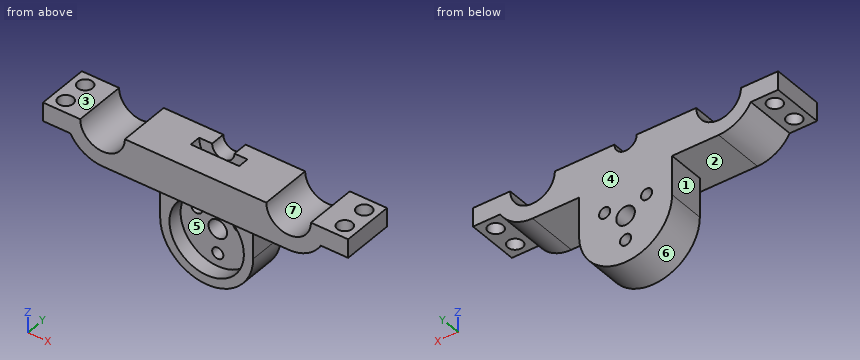
```python
from build123d import *

# Parameters (mm, degrees)
BOSS_EXTRUDE1_DEPTH     = 14
CUT_EXTRUDE1_DEPTH      = 45.463468151
CUT_EXTRUDE1_DEPTH_BACK = 45.463468151
SKETCH4_R               = 2
SKETCH5_W               = 9.30871577
SKETCH5_H               = 4.044371358
BOSS_EXTRUDE2_DEPTH     = 7
CUT_EXTRUDE2_START      = 1.5
SKETCH6_R               = 6.5
CUT_EXTRUDE2_DEPTH      = 1.5
BOSS_EXTRUDE3_DEPTH     = 10
SKETCH8_R               = 10
CUT_EXTRUDE3_DEPTH      = 4
SKETCH9_R               = 2.5
CUT_EXTRUDE4_DEPTH      = 54.235326617
SKETCH10_R              = 1.5
CUT_EXTRUDE5_DEPTH      = 54.235326617


with BuildPart() as part:
    # Sketch2 → Boss-Extrude1 (new body)
    with BuildSketch(Plane(origin=(0, 0, 0), x_dir=(1, 0, 0), z_dir=(0, 1, 0))):
        with BuildLine():
            Line((-3, 0), (-19, 0))
            ThreePointArc((-19, 0), (-25, 6), (-31, 0))
            Line((-31, 0), (-41, 0))
            Line((-41, 0), (-41, 5))
            Line((-41, 5), (-33.660254038, 5))
            ThreePointArc((-33.660254038, 5), (-30, 8.660254038), (-25, 10))
            Line((-25, 10), (25, 10))
            ThreePointArc((25, 10), (30, 8.660254038), (33.660254038, 5))
            Line((33.660254038, 5), (41, 5))
            Line((41, 5), (41, 0))
            Line((41, 0), (31, 0))
            ThreePointArc((31, 0), (25, 6), (19, 0))
            Line((19, 0), (3, 0))
            ThreePointArc((3, 0), (0, 3), (-3, 0))
        make_face()
    extrude(amount=BOSS_EXTRUDE1_DEPTH)

    # Sketch4 → Cut-Extrude1 (cut, two sides: drawn at the far end of the back side and taken through both)
    with BuildSketch(Plane.XY.offset(-CUT_EXTRUDE1_DEPTH_BACK)):
        with Locations((-37.5, 10.5)):
            Circle(SKETCH4_R)
        with Locations((-37.5, 3.5)):
            Circle(SKETCH4_R)
        with Locations((37.5, 10.5)):
            Circle(SKETCH4_R)
        with Locations((37.5, 3.5)):
            Circle(SKETCH4_R)
    extrude(amount=CUT_EXTRUDE1_DEPTH + CUT_EXTRUDE1_DEPTH_BACK, mode=Mode.SUBTRACT)

    # Sketch5 → Boss-Extrude2 (add)
    with BuildSketch(Plane.XZ):
        with Locations((-0.028958253, -2.022185679)):
            Rectangle(SKETCH5_W, SKETCH5_H)
    extrude(amount=-BOSS_EXTRUDE2_DEPTH)

    # Sketch6 → Cut-Extrude2 (cut, symmetric)
    with BuildSketch(Plane(origin=(0, 7, 0), x_dir=(1, 0, 0), z_dir=(0, 1, 0)).offset(CUT_EXTRUDE2_START)):
        Circle(SKETCH6_R)
    extrude(amount=CUT_EXTRUDE2_DEPTH, both=True, mode=Mode.SUBTRACT)

    # Sketch7 → Boss-Extrude3 (add)
    with BuildSketch(Plane(origin=(0, 14, 0), x_dir=(1, 0, 0), z_dir=(0, 1, 0))):
        with BuildLine():
            Line((-12.5, 20.5), (-12.5, 10))
            Line((-12.5, 10), (12.5, 10))
            Line((12.5, 10), (12.5, 20.5))
            ThreePointArc((12.5, 20.5), (0, 33), (-12.5, 20.5))
        make_face()
    extrude(amount=-BOSS_EXTRUDE3_DEPTH)

    # Sketch8 → Cut-Extrude3 (cut)
    with BuildSketch(Plane.XZ.offset(-4)):
        with Locations(Location((0, -20.5, 0), (0, 0, 270))):
            Circle(SKETCH8_R)
    extrude(amount=-CUT_EXTRUDE3_DEPTH, mode=Mode.SUBTRACT)

    # Sketch9 → Cut-Extrude4 (cut, through all)
    with BuildSketch(Plane.XZ.offset(-8)):
        with Locations(Location((0, -20.5, 0), (0, 0, 270))):
            Circle(SKETCH9_R)
    extrude(amount=-CUT_EXTRUDE4_DEPTH, mode=Mode.SUBTRACT)

    # Sketch10 → Cut-Extrude5 (cut, through all)
    with BuildSketch(Plane.XZ.offset(-8)):
        with Locations(Location((0, -27, 0), (0, 0, 270))):
            Circle(SKETCH10_R)
        with Locations(Location((-5.629165125, -17.25, 0), (0, 0, 270))):
            Circle(SKETCH10_R)
        with Locations(Location((5.629165125, -17.25, 0), (0, 0, 270))):
            Circle(SKETCH10_R)
    extrude(amount=-CUT_EXTRUDE5_DEPTH, mode=Mode.SUBTRACT)


solid = part.part
```
The model under review builds one solid part; all positions refer to its coordinate system, in mm. Face numbers are marked on the shaded views. A direction names the side the tool comes from. Round coordinates to 2 decimals unless told otherwise and drop trailing zeros. Write each loop counter-clockwise with the first axis right and the second up, starting at its lowest first coordinate (ties: lowest second). Pieces come first, ordered by that corner, then holes. Notation, with made-up numbers: (-16.5, -35) - (12.5, -35) arc R28 ccw to (12.5, 0) - close; hole circle Ø6 at (50.25, -12.5). An arc over 180 degrees is marked (long way). Answer as CSV lines item,"result". Start each with the question number.
(1) Draft analysis for pull direction Z (two halves, no side actions). For the marked faces 4, 5, 6 and 7, state which applies: pulls with the +Z half, pulls with the -Z half, needs draft (parallel to the pull), parting line crosses it, or undercut.
(2) We need section B-B on z = -16.5. State the section outline as (x, y) points, plus the area to 3 significant figures.
(3) For the marked faces 1, 2 and 3, list the 3-axis set-ups (+Z, -Z, +X, -X, +Y, -Y) from which the entire face can be reached by the end or side of a thin tool; tool diameter is ignored.
(4) We need section D-D on x = 0. State the section outline as (y, z) points.
(5) We need section A-A on x = -37.5. State the section outline as (y, z) points, plus the area to 3 significant figures.
(6) For pin 1 Ø2.5 at (x, y) = (-37.5, 3.5) entering from -Z; pin 2 Ø7 at (x, z) = (-3, -19) entering from -Y; pin 3 Ø3.5 at (x, z) = (1.5, -4) entering from -Y; pin 4 Ø2 at (y, z) = (4, -20.5) entering from +X, all flat-tipped, find the tip position at first contact; note any pin that passes through.
(7) We need section C-C on z = -27. State the section outline as (x, y) points, plus the area to 3 significant figures.
(8) To check wall thickness, follow line 1 (X direction, y = 10, z = -17.25); line 2 (Y direction, x = 37.5, z = -1.45); line 3 (X direction, y = 10.5, z = -1.2). State the ranges of each line that lie inside material, in increasing order.
Worked answers:
1,face 4,"needs draft"
1,face 5,"undercut"
1,face 6,"pulls with the -Z half"
1,face 7,"pulls with the +Z half"
2,outline,"(-12.5, 4) - (-9.17, 4) - (-9.17, 8) - (-6.93, 8) - (-6.93, 14) - (-12.5, 14) - close; (-4.33, 8) - (4.33, 8) - (4.33, 14) - (-4.33, 14) - close; (6.93, 8) - (9.17, 8) - (9.17, 4) - (12.5, 4) - (12.5, 14) - (6.93, 14) - close"
2,area,"146 mm²"
3,face 1,"-Z, -X, +Y, -Y"
3,face 2,"-Z, -Y"
3,face 3,"+Z, +X, -X, +Y, -Y"
4,outline,"(0, -10) - (4, -10) - (4, -10.5) - (8, -10.5) - (8, -18) - (14, -18) - (14, -3) - (10, -3) - (10, -6.5) - (7, -6.5) - (7, 0) - (0, 0) - close; (4, -33) - (14, -33) - (14, -28.5) - (8, -28.5) - (8, -30.5) - (4, -30.5) - close; (8, -25.5) - (14, -25.5) - (14, -23) - (8, -23) - close"
5,outline,"(0, -5) - (1.5, -5) - (1.5, 0) - (0, 0) - close; (5.5, -5) - (8.5, -5) - (8.5, 0) - (5.5, 0) - close; (12.5, -5) - (14, -5) - (14, 0) - (12.5, 0) - close"
5,area,"30.0 mm²"
6,pin 1,"through"
6,pin 2,"y = 8"
6,pin 3,"y = 0"
6,pin 4,"x = 12.5"
7,outline,"(-10.68, 4) - (-7.6, 4) - (-7.6, 8) - (-1.5, 8) - (-1.5, 14) - (-10.68, 14) - close; (1.5, 8) - (7.6, 8) - (7.6, 4) - (10.68, 4) - (10.68, 14) - (1.5, 14) - close"
7,area,"135 mm²"
8,line 1,"-12.5 to -7.13, -4.13 to 4.13, 7.13 to 12.5"
8,line 2,"0 to 1.5, 5.5 to 8.5, 12.5 to 14"
8,line 3,"-41 to -39.5, -35.5 to -30.88, -19.12 to -2.75, 2.75 to 19.12, 30.88 to 35.5, 39.5 to 41"
